from build123d import *

# Parameters (mm, degrees)
F0_W     = 25.4
F0_H     = 25.4
F1_DEPTH = 25.4
F2_R     = 9.525
F3_DEPTH = 19.05
F4_R     = 6.35
F5_DEPTH = 6.351


with BuildPart() as f1:
    # F0 (on Top) → F1 (new body)
    with BuildSketch(Plane.XY):
        with Locations((-3.576601, -18.135061)):
            Rectangle(F0_W, F0_H)
    extrude(amount=F1_DEPTH)

    # F2 (on face) → F3 (cut)
    with BuildSketch(Plane.XY.offset(25.4)):
        with Locations((-3.576601, -18.135061)):
            Circle(F2_R)
    extrude(amount=-F3_DEPTH, mode=Mode.SUBTRACT)

    # F4 (on face) → F5 (cut, through all)
    with BuildSketch(Plane.XY.offset(6.35)):
        with Locations((-3.576601, -18.135061)):
            Circle(F4_R)
    extrude(amount=-F5_DEPTH, mode=Mode.SUBTRACT)


solid = f1.part
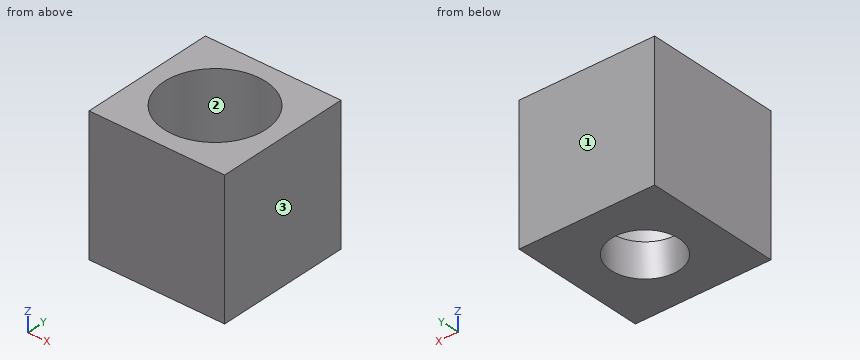
Input: part model. Units: mm. Frame: model coordinates. Face numbers are marked on the shaded views. Coordinates: 2 decimals unless noted, no trailing zeros. Loops run counter-clockwise (first coordinate to the right, second up) from the corner with the lowest first, then second, coordinate; pieces in that order, holes last. Notation, with made-up numbers: (58.5, 86.5) -> (70.5, 86.5) arc R21 cw to (70.5, 103.5) -> close; hole circle Ø5 at (25.25, 88). An arc over 180 degrees is marked (long way). One line per item, written item: value.
(1) Pin query (flat end, axial travel): pin 1 Ø5.5 at (x, y) = (-4.5, -14) entering from +Z; pin 2 Ø11.5 at (x, y) = (-3.58, -18.14) entering from -Z. Return the tip coordinate at first contact, or that it passes through.
Answer below:
pin 1: stops at z = 6.35
pin 2: passes through
(2) Ray query, line 1 along X through (y, z) = (-26.25, 22); line 2 along Z through (x, y) = (-11.75, -21); line 3 along X through (y, z) = (-17, 17.5). Return the intervals inside material, ascending.
Answer below:
line 1: x = -16.28 to -8.56, 1.41 to 9.12
line 2: z = 0 to 6.35
line 3: x = -16.28 to -13.03, 5.88 to 9.12
(3) Cut plane A-A (x = -1.25). Output: boundary loops of the cut face in (y, z).
Answer below:
outline: (-30.84, 0) -> (-24.04, 0) -> (-24.04, 6.35) -> (-27.37, 6.35) -> (-27.37, 25.4) -> (-30.84, 25.4) -> close; (-12.23, 0) -> (-5.44, 0) -> (-5.44, 25.4) -> (-8.9, 25.4) -> (-8.9, 6.35) -> (-12.23, 6.35) -> close
(4) Draft query along Y for the marked faces 1, 2 and 3. Return one class per face: pulls with the +Y half, pulls with the -Y half, needs draft (parallel to the pull), parting line crosses it, or undercut.
Answer below:
face 1: pulls with the +Y half
face 2: undercut
face 3: needs draft
(5) Cut plane D-D (x = 3.5). Output: boundary loops of the cut face in (y, z).
Answer below:
outline: (-30.84, 0) -> (-5.44, 0) -> (-5.44, 25.4) -> (-11.76, 25.4) -> (-11.76, 6.35) -> (-24.51, 6.35) -> (-24.51, 25.4) -> (-30.84, 25.4) -> close
(6) Cut plane C-C (z = 7.25). Output: boundary loops of the cut face in (x, y) (3 decimals), then the cut area to 3 significant figures.
Answer below:
outline: (-16.277, -30.835) -> (9.123, -30.835) -> (9.123, -5.435) -> (-16.277, -5.435) -> close; hole circle Ø19.05 at (-3.577, -18.135)
area: 360 mm2
(7) Cut plane B-B (y = -13.25). Output: boundary loops of the cut face in (x, z), then the cut area to 3 significant figures.
Answer below:
outline: (-16.28, 0) -> (-7.63, 0) -> (-7.63, 6.35) -> (-11.75, 6.35) -> (-11.75, 25.4) -> (-16.28, 25.4) -> close; (0.48, 0) -> (9.12, 0) -> (9.12, 25.4) -> (4.6, 25.4) -> (4.6, 6.35) -> (0.48, 6.35) -> close
area: 282 mm2
